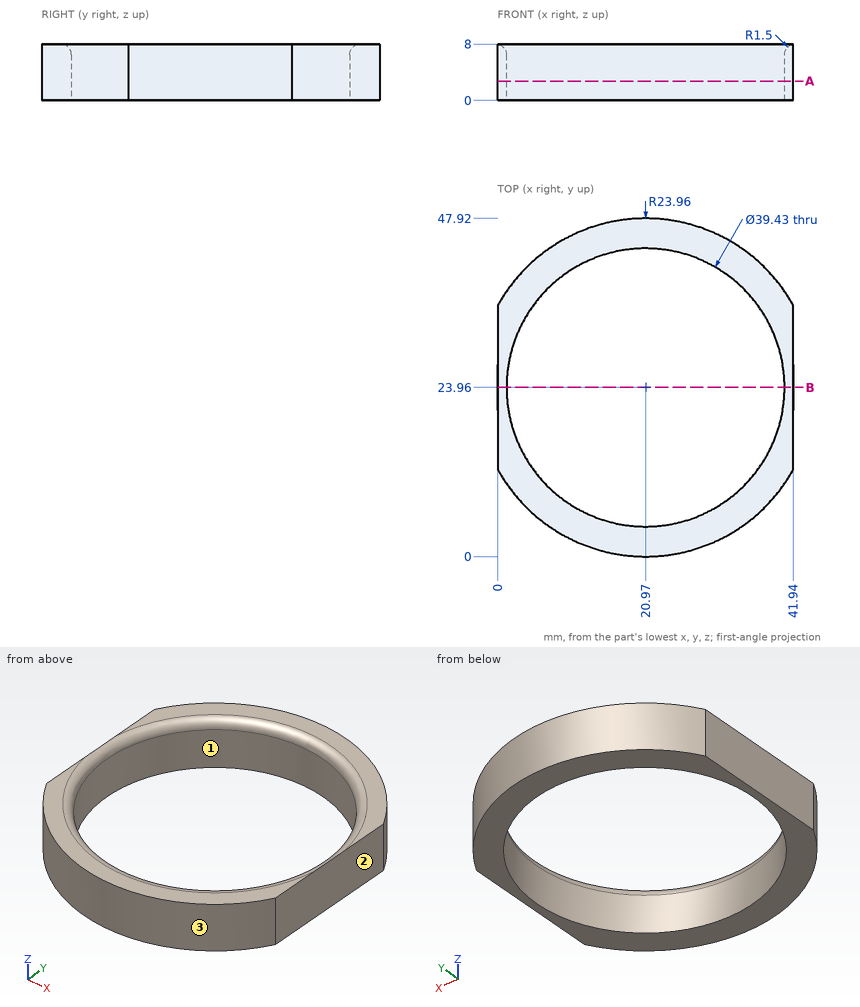
The drawing under review shows one solid part. Ordinate dimensions are in mm from its lowest x, y, z. Coordinates: 2 decimals unless noted, no trailing zeros. Order: outer loops, then holes, each group sorted by start corner. A loop starts at its lowest first (then second) coordinate and runs counter-clockwise, first axis right, second up. Notation, with made-up numbers: (46, 68.5) -> (65, 68.5) arc R14 cw to (65, 86.5) -> close; hole circle Ø11 at (-14, 8). An arc over 180 degrees is marked (long way). Answer in a Markdown table with one row per item. Add a question column.
Item 1: Clearance check with flat-ended pins moving along their axes: pin 1 (1 mm diameter, centred on y = 39.5, z = 4.5, fed in from +X); pin 2 (4 mm diameter, centred on x = 28.5, z = 3.5, fed in from -Y); pin 3 (3 mm diameter, centred on x = 13.5, z = 5, fed in from +Y). State where each tip first meets the part, or that it passes through.
Item 2: We need section B-B on y = 23.96. Write out the cut boundary in (x, z) (3 decimals), plus the area to 3 significant figures.
Item 3: Mouldability with a two-part tool opening along Y and no side actions: class the marked faces 1, 2 and 3 as +Y half, -Y half, draft (parallel to the pull), parting line (faces both ways), or undercut.
Item 4: To check wall thickness, follow probe 1 along X at (y, z) = (24, 4.5); probe 2 along X at (y, z) = (29.5, 5.5); probe 3 along Y at (x, z) = (16, 5.75). State the ranges of each line that lie inside material, in increasing order.
Item 5: We need section A-A on z = 2.75. Write out the cut boundary in (x, y) (3 decimals).
Final values:
| question | item | result |
|---|---|---|
| 1 | pin 1 | stops at x = 39.62 |
| 1 | pin 2 | stops at y = 0.65 |
| 1 | pin 3 | stops at y = 47.16 |
| 2 | outline | (0, 0) -> (1.255, 0) -> (1.255, 6.5) arc R1.5 ccw to (0, 7.98) -> close; (40.685, 0) -> (41.94, 0) -> (41.94, 7.98) arc R1.5 ccw to (40.685, 6.5) -> close |
| 2 | area | 19.1 mm2 |
| 3 | face 1 | undercut |
| 3 | face 2 | draft |
| 3 | face 3 | -Y half |
| 4 | probe 1 | x = 0 to 1.26, 40.68 to 41.94 |
| 4 | probe 2 | x = 0 to 2.05, 39.89 to 41.94 |
| 4 | probe 3 | y = 0.52 to 4.88, 43.04 to 47.4 |
| 5 | outline | (0, 12.369) arc R23.96 ccw to (41.94, 12.369) -> (41.94, 35.551) arc R23.96 ccw to (0, 35.551) -> close; hole circle Ø39.43 at (20.97, 23.96) |
